The figure shows three views and two pictorial views of one solid part (mm, origin at its lowest corner). Answer the questions. Coordinates: 2 decimals unless noted, no trailing zeros. Write each loop counter-clockwise with the first axis right and the second up, starting at its lowest first coordinate (ties: lowest second). Pieces come first, ordered by that corner, then holes.
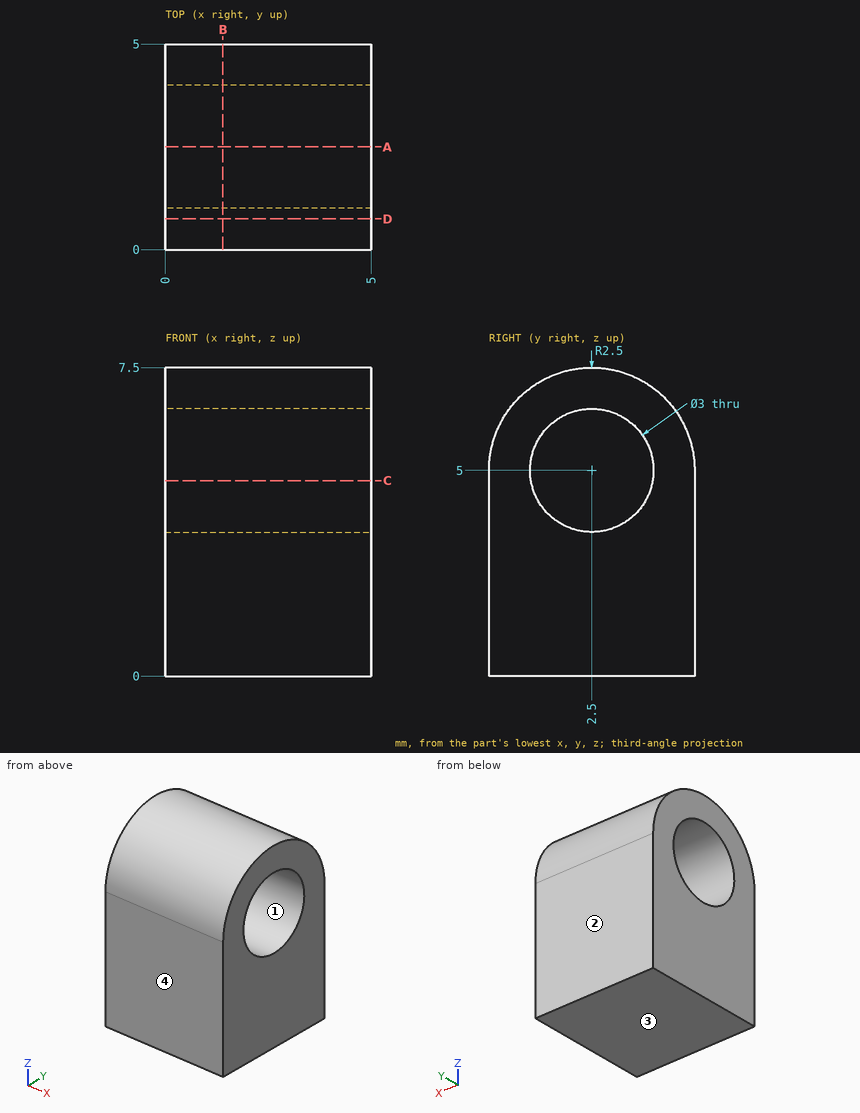
Item 1: The part is cut by section A-A (y = 2.5). Give the vertices of the cut face in (x, z).
Item 2: The part is cut by section B-B (x = 1.4). Give the vertices of the cut face in (y, z).
Item 3: Find the intervals of material crossed by probe 1 along Y at (x, z) = (2, 5); probe 2 along Z at (x, y) = (1, 1.5); probe 3 along Z at (x, y) = (3.4, 1.2), in increasing order.
Item 4: The part is cut by section C-C (z = 4.75). Give the vertices of the cut face in (x, y), and give its area (3 significant figures).
Item 5: The part is cut by section D-D (y = 0.75). Give the vertices of the cut face in (x, z).
Item 6: Given pin 1 (2 mm diameter, centred on x = 3, y = 1, fed in from +Z), flat-ended and moving along its own axis, determine where the tip first touches the part or whether it passes through.
Item 7: Determine the mould class of the marked faces 1, 2, 3 and 4 for opening direction Y: +Y half, -Y half, draft (parallel to the pull), parting line (faces both ways), or undercut.
Answer:
1. outline: (0, 0) - (5, 0) - (5, 3.5) - (0, 3.5) - close; (0, 6.5) - (5, 6.5) - (5, 7.5) - (0, 7.5) - close
2. outline: (0, 0) - (5, 0) - (5, 5) arc R2.5 ccw to (0, 5) - close; hole circle Ø3 at (2.5, 5)
3. probe 1: y = 0 to 1, 4 to 5
3. probe 2: z = 0 to 3.88, 6.12 to 7.29
3. probe 3: z = 0 to 4.25, 5.75 to 7.14
4. outline: (0, 0) - (5, 0) - (5, 1.02) - (0, 1.02) - close; (0, 3.98) - (5, 3.98) - (5, 5) - (0, 5) - close
4. area: 10.2 mm2
5. outline: (0, 0) - (5, 0) - (5, 6.79) - (0, 6.79) - close
6. pin 1: stops at z = 7.45
7. face 1: undercut
7. face 2: +Y half
7. face 3: draft
7. face 4: -Y half
